Geometry check sheet. Reference: the model listing, model coordinates, mm. A direction names the side the tool comes from. Round coordinates to 2 decimals unless told otherwise and drop trailing zeros. Order: outer loops, then holes, each group sorted by start corner. A loop starts at its lowest first (then second) coordinate and runs counter-clockwise, first axis right, second up.
(1) Sectioned sample at A-A (z = 3). Give the number of separate pieces and of enclosed holes in the cut face, plus the area to 3 significant figures.
(2) Set-up check for faces 1 (the face through (18, -13, 11)), 2 (the face through (-7.63, 9.98, 3.37)), 3 (the face through (-9, -14, 3)), 4 (the face through (4, -14, 3)), 5 (the face through (-11, 0, 1)): record each of +Z, -Z, +X, -X, +Y, -Y from which the full face is reachable in a straight line by a thin tool's end or side.
(3) Sectioned sample at D-D (y = -13). Record the boundary of the cut face in (x, z).
(4) Release check for a two-part mould opening along Y. For faces 6 (the face through (6, 13, 5.3)), 7 (the face through (-7, -10, 1.5)) record: +Y half, -Y half, draft (parallel to the pull), parting line (faces both ways), or undercut.
(5) Sectioned sample at C-C (x = -7). Record the boundary of the cut face in (y, z), plus the area to 3 significant figures.
(6) Sectioned sample at B-B (y = 0). Record the boundary of the cut face in (x, z).
(7) Material ranges on line 1 along Y through (x, z) = (-7, 3.4); line 2 along X through (y, z) = (-10.5, 3.4); line 3 along Y through (x, z) = (0, 1.05), recorded low to high.
(8) Go/stop test with flat-tipped pins: pin 1 (1.3 mm diameter, centred on x = -7, y = 10.47, fed in from +Z); pin 2 (1.8 mm diameter, centred on x = -7, y = 10.5, fed in from +Z); pin 3 (1.9 mm diameter, centred on y = 12, z = 3.5, fed in from -X). Record where each tip stops, or that it passes through.
from build123d import *

# Parameters (mm, degrees)
SKETCH023_W      = 12
SKETCH023_H      = 4.8
PAD011_DEPTH     = 30
SKETCH026_W      = 8.3
SKETCH026_H      = 4.2
PAD014_DEPTH     = 30
BOX014_W         = 15
BOX014_H         = 15
BOX014_DEPTH     = 10
SKETCH025_W      = 8.2
SKETCH025_H      = 4.2
PAD013_DEPTH     = 30
SKETCH020_R      = 1
PAD007_DEPTH     = 20
SKETCH021_R      = 1
PAD008_DEPTH     = 11
SKETCH022_R      = 0.8
PAD009_DEPTH     = 5.3
MIRROREDSKETCH_R = 0.8
PAD010_DEPTH     = 5.3
PAD018_DEPTH     = 3
ARRAY007_X_COUNT = 2
ARRAY007_X_PITCH = 70
SKETCH_R         = 8.5
PAD_DEPTH        = 1.5
BOX013_W         = 30
BOX013_H         = 34
BOX013_DEPTH     = 21


with BuildPart() as body006:
    # Sketch023 → Pad011 (new body)
    with BuildSketch(Plane.XZ):
        with Locations((-29.8, 14.9)):
            Rectangle(SKETCH023_W, SKETCH023_H)
    extrude(amount=PAD011_DEPTH)


with BuildPart() as body:
    # Sketch026 → Pad014 (new body)
    with BuildSketch(Plane.XZ):
        with Locations((11.75, 14.6)):
            Rectangle(SKETCH026_W, SKETCH026_H)
    extrude(amount=PAD014_DEPTH)


with BuildPart() as camera_hole_extract_cube:
    # Box014 → Box014 (new body)
    with BuildSketch(Plane(origin=(-7.5, -7.5, 1), x_dir=(1, 0, 0), z_dir=(0, 0, 1))):
        with Locations((7.5, 7.5)):
            Rectangle(BOX014_W, BOX014_H)
    extrude(amount=BOX014_DEPTH)


with BuildPart() as extract_fusion002:
    # Sketch025 → Pad013 (new body)
    with BuildSketch(Plane.XZ):
        with Locations((-0.9, 14.6)):
            Rectangle(SKETCH025_W, SKETCH025_H)
    extrude(amount=PAD013_DEPTH)

    # Fusion010: union Body006, Body, camera hole extract cube
    add(body006.part)
    add(body.part)
    add(camera_hole_extract_cube.part)


with BuildPart() as level3_body:
    # Sketch020 → Pad007 (new body)
    with BuildSketch(Plane.XY):
        with BuildLine():
            Line((-56, 13), (-56, 9))
            Line((-56, 9), (-47.5, 9))
            Line((-47.5, 9), (-47.5, 17))
            Line((-47.5, 17), (26, 17))
            ThreePointArc((29, 14), (28.12132, 16.12132), (26, 17))
            Line((29, 8.86), (29, 14))
            ThreePointArc((29, 8.86), (29.146447, 8.506447), (29.5, 8.36))
            Line((29.5, 8.36), (31.5, 8.36))
            ThreePointArc((33, 6.86), (32.56066, 7.92066), (31.5, 8.36))
            Line((33, -6.86), (33, 6.86))
            ThreePointArc((31.5, -8.36), (32.56066, -7.92066), (33, -6.86))
            Line((29.5, -8.36), (31.5, -8.36))
            ThreePointArc((29.5, -8.36), (29.146447, -8.506447), (29, -8.86))
            Line((29, -8.86), (29, -14))
            ThreePointArc((26, -17), (28.12132, -16.12132), (29, -14))
            Line((-47.5, -17), (26, -17))
            Line((-47.5, -9), (-47.5, -17))
            Line((-56, -9), (-47.5, -9))
            Line((-56, -9), (-56, -13))
            ThreePointArc((-56, -13), (-54.535534, -16.535534), (-51, -18))
            Line((31, -18), (-51, -18))
            ThreePointArc((31, -18), (38.238337, 0), (31, 18))
            Line((-51, 18), (31, 18))
            ThreePointArc((-51, 18), (-54.535534, 16.535534), (-56, 13))
        make_face()
        with Locations((-52, -14.3)):
            Circle(SKETCH020_R, mode=Mode.SUBTRACT)
        with Locations((31.5, 11.4)):
            Circle(SKETCH020_R, mode=Mode.SUBTRACT)
        with Locations((31.5, -11.4)):
            Circle(SKETCH020_R, mode=Mode.SUBTRACT)
        with Locations((-52, 14.3)):
            Circle(SKETCH020_R, mode=Mode.SUBTRACT)
    extrude(amount=PAD007_DEPTH)


with BuildPart() as level2_body:
    # Sketch021 → Pad008 (new body)
    with BuildSketch(Plane.XY):
        with BuildLine():
            Line((-56, 13), (-56, 9))
            Line((-56, 9), (-36.211556, 9))
            ThreePointArc((-36.211556, 9), (-35.354856, 9.354856), (-35, 10.211556))
            Line((-35, 10.211556), (-35, 17))
            Line((-35, 17), (17, 17))
            Line((17, 17), (17, 11))
            ThreePointArc((17, 11), (17.585786, 9.585786), (19, 9))
            Line((19, 9), (31.5, 9))
            ThreePointArc((33, 7.5), (32.56066, 8.56066), (31.5, 9))
            Line((33, -7.5), (33, 7.5))
            ThreePointArc((31.5, -9), (32.56066, -8.56066), (33, -7.5))
            Line((19, -9), (31.5, -9))
            ThreePointArc((19, -9), (17.585786, -9.585786), (17, -11))
            Line((17, -17), (17, -11))
            Line((-35, -17), (17, -17))
            Line((-35, -10.211556), (-35, -17))
            ThreePointArc((-35, -10.211556), (-35.354856, -9.354856), (-36.211556, -9))
            Line((-56, -9), (-36.211556, -9))
            Line((-56, -9), (-56, -13))
            ThreePointArc((-56, -13), (-54.535534, -16.535534), (-51, -18))
            Line((31, -18), (-51, -18))
            ThreePointArc((31, -18), (38.238337, 0), (31, 18))
            Line((-51, 18), (31, 18))
            ThreePointArc((-51, 18), (-54.535534, 16.535534), (-56, 13))
        make_face()
        with Locations((-39.037737, 11.5)):
            Circle(SKETCH021_R, mode=Mode.SUBTRACT)
        with Locations((-39.037737, -11.5)):
            Circle(SKETCH021_R, mode=Mode.SUBTRACT)
        with Locations((19.215181, 11.5)):
            Circle(SKETCH021_R, mode=Mode.SUBTRACT)
        with Locations((19.215181, -11.5)):
            Circle(SKETCH021_R, mode=Mode.SUBTRACT)
    extrude(amount=PAD008_DEPTH)


with BuildPart() as level_1_body:
    # Sketch022 → Pad009 (new body)
    with BuildSketch(Plane.XY):
        with BuildLine():
            Line((-9, 18), (-9, 10.470701))
            ThreePointArc((-9, 10.470701), (-7, 8.470701), (-5, 10.470701))
            Line((-5, 17), (-5, 10.470701))
            Line((-5, 17), (4, 17))
            Line((4, 17), (4, 10.5))
            ThreePointArc((4, 10.5), (6, 8.5), (8, 10.5))
            Line((8, 18), (8, 10.5))
            Line((8, 18), (-9, 18))
        make_face()
        with Locations((-7, 10.470701)):
            Circle(SKETCH022_R, mode=Mode.SUBTRACT)
        with Locations((6, 10.5)):
            Circle(SKETCH022_R, mode=Mode.SUBTRACT)
    extrude(amount=PAD009_DEPTH)


with BuildPart() as level_1_mirror:
    # MirroredSketch → Pad010 (new body)
    with BuildSketch(Plane.XY):
        with BuildLine():
            Line((-9, -18), (-9, -10.470701))
            ThreePointArc((-5, -10.470701), (-7, -8.470701), (-9, -10.470701))
            Line((-5, -17), (-5, -10.470701))
            Line((-5, -17), (4, -17))
            Line((4, -17), (4, -10.5))
            ThreePointArc((8, -10.5), (6, -8.5), (4, -10.5))
            Line((8, -18), (8, -10.5))
            Line((8, -18), (-9, -18))
        make_face()
        with Locations((-7, -10.470701)):
            Circle(MIRROREDSKETCH_R, mode=Mode.SUBTRACT)
        with Locations((6, -10.5)):
            Circle(MIRROREDSKETCH_R, mode=Mode.SUBTRACT)
    extrude(amount=PAD010_DEPTH)


with BuildPart() as attach_body:
    # Sketch030 → Pad018 (new body)
    with BuildSketch(Plane.XY):
        with BuildLine():
            Line((-49.771311, 17), (-49.771311, 32))
            ThreePointArc((-39.771311, 32), (-44.771311, 37), (-49.771311, 32))
            Line((-39.771311, 17), (-39.771311, 32))
            Line((-49.771311, 17), (-39.771311, 17))
        make_face()
        with BuildLine():
            Line((-46.571311, 32), (-46.571311, 22))
            ThreePointArc((-46.571311, 22), (-44.771311, 20.2), (-42.971311, 22))
            Line((-42.971311, 32), (-42.971311, 22))
            ThreePointArc((-42.971311, 32), (-44.771311, 33.8), (-46.571311, 32))
        make_face(mode=Mode.SUBTRACT)
    extrude(amount=PAD018_DEPTH)


with BuildPart() as attachment_array:
    # Part__Mirroring001: instance of attach body
    add(attach_body.part.mirror(Plane(origin=(0, 0, 0), x_dir=(1, 0, 0), z_dir=(0, 1, 0))))

    # Fusion012: union attach body
    add(attach_body.part)

    # Array007 X: attachment array ×2


with BuildPart() as attachment_array_1:
    add(attachment_array.part)
    with Locations(*[(i * ARRAY007_X_PITCH, 0, 0) for i in range(1, ARRAY007_X_COUNT)]):
        add(attachment_array.part)


with BuildPart() as obj1:
    # Sketch → Pad (new body)
    with BuildSketch(Plane.XY):
        with BuildLine():
            Line((-56, 13), (-56, -13))
            ThreePointArc((-56, -13), (-54.535534, -16.535534), (-51, -18))
            Line((31, -18), (-51, -18))
            ThreePointArc((31, -18), (38.238337, 0), (31, 18))
            Line((-51, 18), (31, 18))
            ThreePointArc((-51, 18), (-54.535534, 16.535534), (-56, 13))
        make_face()
        Circle(SKETCH_R, mode=Mode.SUBTRACT)
    extrude(amount=PAD_DEPTH)

    # Fusion009: union level3 body, level2 body, level 1 body, level 1 mirror, attachment array
    add(level3_body.part)
    add(level2_body.part)
    add(level_1_body.part)
    add(level_1_mirror.part)
    add(attachment_array_1.part)

    # Cut002005: cut extract fusion002
    add(extract_fusion002.part, mode=Mode.SUBTRACT)


with BuildPart() as common:
    # Box013 → Box013 (new body)
    with BuildSketch(Plane(origin=(-11, -17, 0), x_dir=(1, 0, 0), z_dir=(0, 0, 1))):
        with Locations((15, 17)):
            Rectangle(BOX013_W, BOX013_H)
    extrude(amount=BOX013_DEPTH)

    # Common: intersect obj1
    add(obj1.part, mode=Mode.INTERSECT)


solid = common.part
Answer below:
1. separate pieces: 6
1. enclosed holes: 4
1. area: 149 mm2
2. face 1: +Z, +X, -X, +Y, -Y
2. face 2: +Z
2. face 3: +Z, -X, +Y, -Y
2. face 4: +Z, +Y, -Y
2. face 5: +Z, -Z, -X, +Y, -Y
3. outline: (-11, 0) - (19, 0) - (19, 11) - (17, 11) - (17, 1.5) - (8, 1.5) - (8, 5.3) - (4, 5.3) - (4, 1.5) - (-5, 1.5) - (-5, 5.3) - (-9, 5.3) - (-9, 1.5) - (-11, 1.5) - close
4. face 6: draft
4. face 7: undercut
5. outline: (-17, 0) - (-4.82, 0) - (-4.82, 1) - (-7.5, 1) - (-7.5, 1.5) - (-8.47, 1.5) - (-8.47, 5.3) - (-9.67, 5.3) - (-9.67, 1.5) - (-11.27, 1.5) - (-11.27, 5.3) - (-17, 5.3) - close; (4.82, 0) - (17, 0) - (17, 5.3) - (11.27, 5.3) - (11.27, 1.5) - (9.67, 1.5) - (9.67, 5.3) - (8.47, 5.3) - (8.47, 1.5) - (7.5, 1.5) - (7.5, 1) - (4.82, 1) - close
5. area: 86.5 mm2
6. outline: (-11, 0) - (-8.5, 0) - (-8.5, 1.5) - (-11, 1.5) - close; (8.5, 0) - (19, 0) - (19, 1.5) - (8.5, 1.5) - close
7. line 1: y = -17 to -11.27, -9.67 to -8.47, 8.47 to 9.67, 11.27 to 17
7. line 2: x = -9 to -7.8, -6.2 to -5, 4 to 5.2, 6.8 to 8, 17.06 to 19
7. line 3: y = -17 to -8.5, 8.5 to 17
8. pin 1: stops at z = 1.5
8. pin 2: stops at z = 5.3
8. pin 3: stops at x = -9
